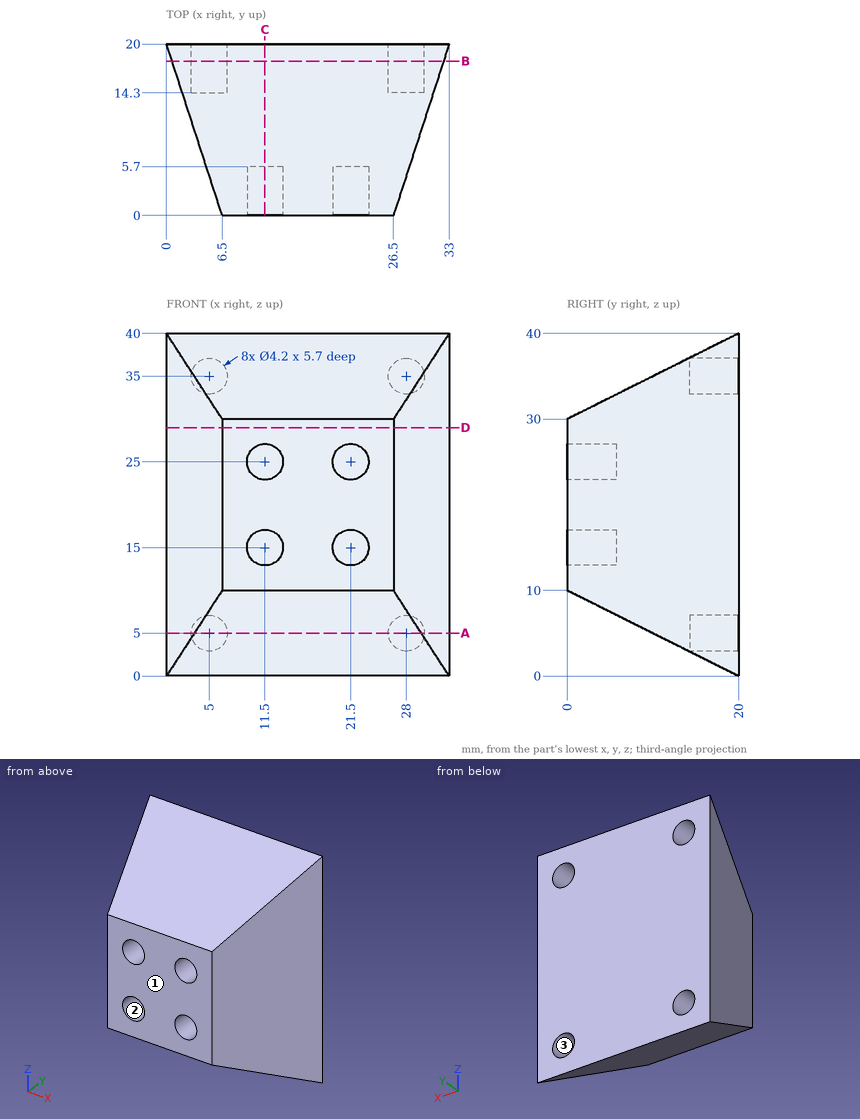
Source: three-view drawing plus pictorial views. Frame: mm from the lowest corner of the part. A direction names the side the tool comes from. Round coordinates to 2 decimals unless told otherwise and drop trailing zeros. Loops run counter-clockwise (first coordinate to the right, second up) from the corner with the lowest first, then second, coordinate; pieces in that order, holes last.
Q1. Section D-D, the plane z = 29. Return loops of the section in (x, y), plus the area to 3 significant figures.
Q2. Section C-C, the plane x = 11.5. Return loops of the section in (y, z).
Q3. Section B-B, the plane y = 18. Return loops of the section in (x, z).
Q4. Ray query, line 1 (Z direction, x = 10, y = 2.25) (3 decimals); line 2 (Y direction, x = 11.5, z = 27); line 3 (Y direction, x = 27.5, z = 5). Return the intervals inside material, ascending.
Q5. Access query for the marked faces 1, 2 and 3. Directions: +Z, -Z, +X, -X, +Y, -Y. A direction counts if a zero-diameter tool reaches every point of the face in a straight line with its end or side. Return the directions, or none.
Q6. Section A-A, the plane z = 5. Return loops of the section in (x, y), plus the area to 3 significant figures.
Q7. First-contact query: P1, Ø3.5, axis at x = 11.5, z = 25, coming from the -Y side; P2, Ø1.3, axis at x = 29, z = 6, coming from the +Y side; P3, Ø6, axis at x = 3.5, y = 6.5, coming from the +Z side; P4, Ø3.5, axis at x = 22, z = 14.5, coming from the -Y side. Flat tips, straight axial feed; report the tip coordinate or a pass-through.
Solutions:
1. outline: (0, 20) - (6.5, 0) - (26.5, 0) - (33, 20) - close
1. area: 530 mm2
2. outline: (0, 10) - (20, 0) - (20, 40) - (0, 30) - (0, 27.1) - (5.7, 27.1) - (5.7, 22.9) - (0, 22.9) - (0, 17.1) - (5.7, 17.1) - (5.7, 12.9) - (0, 12.9) - close
3. outline: (0.65, 1) - (32.35, 1) - (32.35, 39) - (0.65, 39) - close; hole circle Ø4.2 at (5, 5); hole circle Ø4.2 at (5, 35); hole circle Ø4.2 at (28, 5); hole circle Ø4.2 at (28, 35)
4. line 1: z = 8.875 to 13.53, 16.47 to 23.53, 26.47 to 31.125
4. line 2: y = 5.7 to 20
4. line 3: y = 10 to 14.3
5. face 1: +Z, -Z, +X, -X, -Y
5. face 2: -Y
5. face 3: +Y
6. outline: (0, 20) - (3.25, 10) - (29.75, 10) - (33, 20) - (30.1, 20) - (30.1, 14.3) - (25.9, 14.3) - (25.9, 20) - (7.1, 20) - (7.1, 14.3) - (2.9, 14.3) - (2.9, 20) - close
6. area: 250 mm2
7. P1: stops at y = 5.7
7. P2: stops at y = 14.3
7. P3: stops at z = 34.75
7. P4: stops at y = 0
